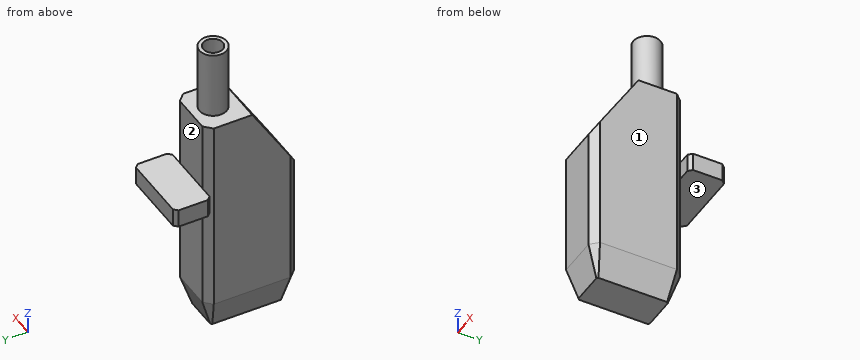
```python
from build123d import *

# Parameters (mm, degrees)
BOSS_EXTRUDE1_DEPTH = 108
SKETCH2_R           = 7.424298736
SKETCH2_R_2         = 5.332436938
BOSS_EXTRUDE2_DEPTH = 37
BOSS_EXTRUDE3_DEPTH = 10
CUT_EXTRUDE1_REACH  = 157.804
BOSS_EXTRUDE5_DEPTH = 17
BOSS_EXTRUDE5_TAPER = 18


with BuildPart() as part:
    # Sketch1 → Boss-Extrude1 (new body)
    with BuildSketch(Plane.XY):
        Polygon((-11, 25), (-15, 21), (-15, -21), (-11, -25), (11, -25), (15, -21), (15, 21), (11, 25), align=None)
    extrude(amount=BOSS_EXTRUDE1_DEPTH)

    # Sketch2 → Boss-Extrude2 (add)
    with BuildSketch(Plane.XY.offset(108)):
        with Locations((0, 13.003641212)):
            Circle(SKETCH2_R)
        with Locations((0, 13.003641212)):
            Circle(SKETCH2_R_2, mode=Mode.SUBTRACT)
    extrude(amount=BOSS_EXTRUDE2_DEPTH)

    # Sketch3 → Boss-Extrude3 (add)
    with BuildSketch(Plane(origin=(0, 0, 70), x_dir=(-1, 0, 0), z_dir=(0, 0, -1))):
        Polygon((-18, 45), (18, 45), (20, 43), (20, 27), (18, 25), (-18, 25), (-20, 27), (-20, 43), align=None)
    extrude(amount=BOSS_EXTRUDE3_DEPTH)

    # Sketch4 → Cut-Extrude1 (cut, up to next)
    with BuildSketch(Plane.ZY.offset(15), mode=Mode.PRIVATE) as cut_extrude1_sk1:
        Polygon((108, 0), (67.685614015, -25), (108, -25), align=None)
    cut_extrude1_tool1 = extrude(cut_extrude1_sk1.sketch, amount=-CUT_EXTRUDE1_REACH, mode=Mode.PRIVATE) & part.part
    add(cut_extrude1_tool1.solids().sort_by_distance((-15, -16.666667, 94.561871))[0], mode=Mode.SUBTRACT)

    # Sketch5 → Boss-Extrude5 (add)
    with BuildSketch(Plane(origin=(-28.517335014, 0, 0), x_dir=(-1, 0, 0), z_dir=(0, 0, -1))):
        Polygon((-43.517335014, 21), (-43.517335014, -21), (-39.517335014, -25), (-17.517335014, -25), (-13.517335014, -21), (-13.517335014, 21), (-17.517335014, 25), (-39.517335014, 25), align=None)
    extrude(amount=BOSS_EXTRUDE5_DEPTH, taper=BOSS_EXTRUDE5_TAPER)


solid = part.part
```
CAD build for the part. Positions are in the model's coordinates, mm. Face numbers are marked on the shaded views. A direction names the side the tool comes from. Round coordinates to 2 decimals unless told otherwise and drop trailing zeros. Order: outer loops, then holes, each group sorted by start corner. A loop starts at its lowest first (then second) coordinate and runs counter-clockwise, first axis right, second up. Notation, with made-up numbers: (28.25, 21) -> (48.25, 21) arc R12 ccw to (48.25, 42) -> close; hole circle Ø10 at (58, 66). An arc over 180 degrees is marked (long way). Write item = value, one per line.
(1) 3-axis set-ups, long thin cutter, end or side, ignore diameter. For the marked faces 1, 2 and 3: which of +Z, -Z, +X, -X, +Y, -Y reach the whole face in a straight line?
Answers follow:
face_1 = +Z, -Z, +X, -Y
face_2 = +Z, +X, -X, +Y
face_3 = -Z, +X, -X, +Y
(2) Cut at A-A (y = 31). Write the cut outline in (x, z), plus the area to 3 significant figures.
Answers follow:
outline = (-20, 60) -> (20, 60) -> (20, 70) -> (-20, 70) -> close
area = 400 mm²
(3) Drill centre lines: L1, parallel to Y at x = 0, z = 133.5; L2, parallel to X at y = 13, z = 30.5; L3, parallel to Y at x = -1.5, z = 132. Where is each one in solid material? Low to high.
Answers follow:
L1 = 5.58 to 7.67, 18.34 to 20.43
L2 = -15 to 15
L3 = 5.73 to 7.89, 18.12 to 20.27
(4) Cut at B-B (z = 126). Write the cut outline in (x, y), plus the area to 3 significant figures.
Answers follow:
outline = circle Ø14.85 at (0, 13); hole circle Ø10.66 at (0, 13)
area = 83.8 mm²
(5) Flat gauge pins, fed straight in: P1, Ø10, axis at x = 8, y = 39, coming from the -Z side; P2, Ø1.5, axis at x = -7, y = 28, coming from the +Z side; P3, Ø21, axis at y = -5, z = 48.5, coming from the -X side. Where does each tip first touch, or does it go through?
Answers follow:
P1 = 60
P2 = 70
P3 = -15
